```python
from build123d import *

# Parameters (mm, degrees)
TAGLIO_ESTRUSIONE1_DEPTH    = 153.019930179
RIPETIZIONECIRCOLARE1_COUNT = 4


with BuildPart() as part:
    # Schizzo1 → Rivoluzione1 (revolve)
    with BuildSketch(Plane(origin=(0, 0, 0), x_dir=(0, 0, -1), z_dir=(1, 0, 0)), mode=Mode.PRIVATE) as rivoluzione1_sk:
        Polygon((-40.820512821, 20), (65.179487179, 20), (65.179487179, 48), (95.179487179, 48), (95.179487179, 62.5), (60.717948718, 62.5), (60.717948718, 80), (40.179487179, 80), (40.179487179, 40.666666667), (25.179487179, 40.666666667), (25.179487179, 48), (5.179487179, 48), (5.179487179, 38), (-20.820512821, 38), (-20.820512821, 48), (-40.820512821, 48), align=None)
    revolve(rivoluzione1_sk.sketch.rotate(Axis((0, 0, 49.025641026), (0, 0, -1)), 90), axis=Axis((0, 0, 49.025641026), (0, 0, -1)))

    # Schizzo2 → Taglio-Estrusione1 (cut, through all)
    with BuildSketch(Plane(origin=(0, 0, -60.717948718), x_dir=(-1, 0, 0), z_dir=(0, 0, -1))):
        with BuildLine():
            ThreePointArc((26.979181982, 65.133507042), (49.851028074, 49.851028074), (65.133507042, 26.979181982))
            Line((65.133507042, 26.979181982), (73.910362601, 30.614674589))
            ThreePointArc((73.910362601, 30.614674589), (56.568542495, 56.568542495), (30.614674589, 73.910362601))
            Line((30.614674589, 73.910362601), (26.979181982, 65.133507042))
        make_face()
    taglio_estrusione1 = extrude(amount=-TAGLIO_ESTRUSIONE1_DEPTH, mode=Mode.SUBTRACT)

    # RipetizioneCircolare1: Taglio-Estrusione1 ×4 about axis
    ripetizionecircolare1_axis = Axis((0, 0, 49.025641026), (0, 0, 1))
    for i in range(1, RIPETIZIONECIRCOLARE1_COUNT):
        add(taglio_estrusione1.rotate(ripetizionecircolare1_axis, i * 360 / RIPETIZIONECIRCOLARE1_COUNT), mode=Mode.SUBTRACT)


solid = part.part
```
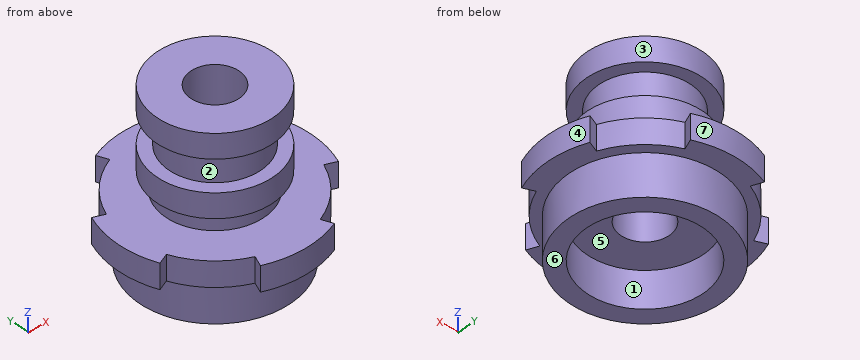
The listing builds one solid part. Answer for the finished solid, in the listing's coordinates (mm). Face numbers are marked on the shaded views. A direction names the side the tool comes from. Round coordinates to 2 decimals unless told otherwise and drop trailing zeros. Write each loop counter-clockwise with the first axis right and the second up, starting at its lowest first coordinate (ties: lowest second). Pieces come first, ordered by that corner, then holes. Notation, with made-up numbers: (-23.5, -20.75) -> (4.5, -20.75) arc R26 cw to (4.5, 12.25) -> close; hole circle Ø11 at (-22, 6.25). An arc over 180 degrees is marked (long way). Write item = value, one per line.
1) For a pull along Y with two mould halves and no side action, classify the marked faces 5, 6 and 7 as released by +Y, released by -Y, zero draft, split by the parting line, or undercut.
Check values:
face_5 = undercut
face_6 = zero draft
face_7 = released by +Y
2) Section D-D on y = 53.5 is taken. Write down the section's boundary in (x, z).
Check values:
outline = (-45.91, -60.72) -> (-32.31, -60.72) -> (-32.31, -95.18) -> (32.31, -95.18) -> (32.31, -60.72) -> (45.91, -60.72) -> (45.91, -40.18) -> (-45.91, -40.18) -> close
3) Given pin 1 (1 mm diameter, centred on x = -57.5, z = -42, fed in from -Y); pin 2 (10 mm diameter, centred on y = 46, z = -58.5, fed in from -X); pin 3 (3 mm diameter, centred on x = 10, z = 3.5, fed in from +Y), each flat-ended and moving along its own axis, determine where each tip first touches the part or whether it passes through.
Check values:
pin_1 = -41.49
pin_2 = -57.35
pin_3 = 37.04
4) Straight lines are drawn through the part: line 1 along Z through (x, y) = (32.5, -28); line 2 along Y through (x, z) = (0, -79.5); line 3 along Z through (x, y) = (-43.5, -36). For each, find the intervals that lie inside material, in ascending order. Write a range as [from, to].
Check values:
line_1 = [-65.18, -40.18], [-25.18, -5.18], [20.82, 40.82]
line_2 = [-62.5, -48], [48, 62.5]
line_3 = [-95.18, -40.18]
5) Which of the six approach directions +Z, -Z, +X, -X, +Y, -Y give full straight-line access (tool end or side, diameter ignored) to the marked faces 1, 2, 3 and 4?
Check values:
face_1 = -Z
face_2 = none
face_3 = +Z
face_4 = +Z, -Z, +X
6) Section C-C on x = 45 is taken. Write down the section's boundary in (y, z), plus the area to 3 significant figures.
Check values:
outline = (-54.27, -60.72) -> (-43.37, -60.72) -> (-43.37, -95.18) -> (-16.7, -95.18) -> (-16.7, -65.18) -> (16.7, -65.18) -> (16.7, -95.18) -> (43.37, -95.18) -> (43.37, -60.72) -> (54.27, -60.72) -> (54.27, -40.18) -> (-54.27, -40.18) -> close; (-16.7, -25.18) -> (16.7, -25.18) -> (16.7, -5.18) -> (-16.7, -5.18) -> close; (-16.7, 20.82) -> (16.7, 20.82) -> (16.7, 40.82) -> (-16.7, 40.82) -> close
area = 5,550 mm²
